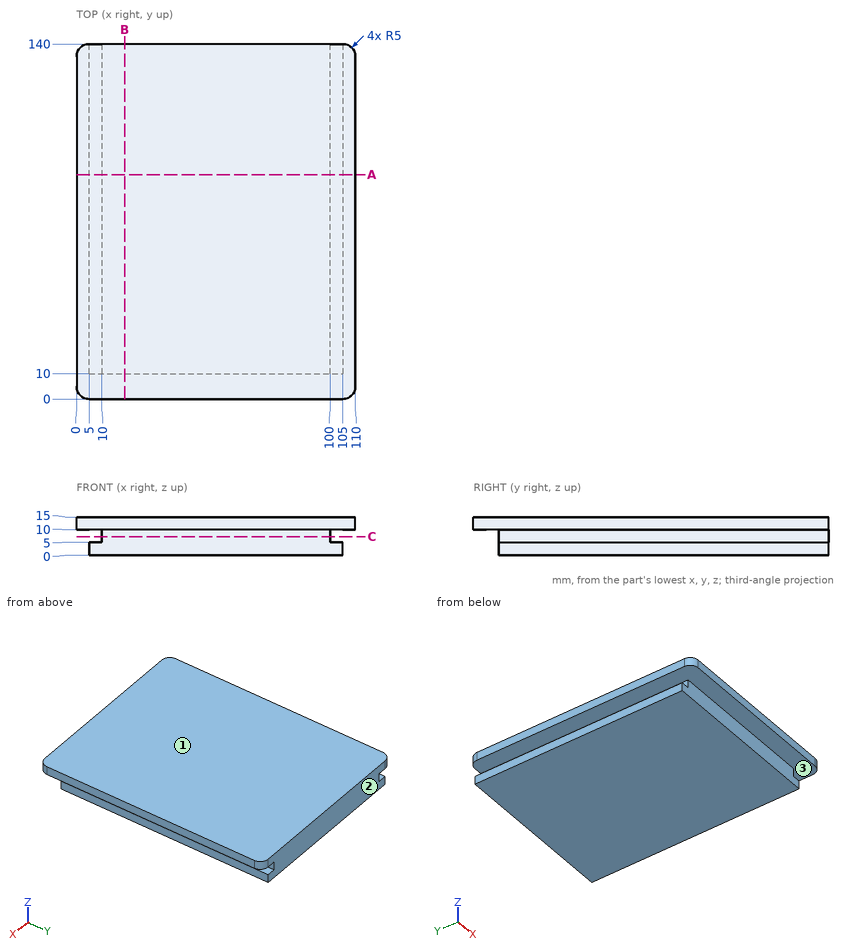
The figure shows three views and two pictorial views of one solid part (mm, origin at its lowest corner). Answer the questions. Coordinates: 2 decimals unless noted, no trailing zeros. Loops run counter-clockwise (first coordinate to the right, second up) from the corner with the lowest first, then second, coordinate; pieces in that order, holes last. Notation, with made-up numbers: (47, 35.25) - (106, 35.25) arc R12 ccw to (106, 57.25) - close; hole circle Ø9 at (55.5, 10). An arc over 180 degrees is marked (long way). Use a Markdown table: item, result. Add a question column.
1) The mould has two halves that part along Z. Classify the marked faces 1, 2 and 3: released by +Z, released by -Z, zero draft, split by the parting line, or undercut.
2) The part is cut by section C-C, the plane z = 7.25. Give the vertices of the cut face in (x, y).
3) Given pin 1 (2.5 mm diameter, centred on y = 85, z = 7.5, fed in from -X); pin 2 (4 mm diameter, centred on y = 68.5, z = 3.5, fed in from -X); pin 3 (1.5 mm diameter, centred on y = 67.5, z = 7, fed in from +X), each flat-ended and moving along its own axis, determine where each tip first touches the part or whether it passes through.
4) The part is cut by section B-B, the plane x = 19. Give the vertices of the cut face in (y, z), and give its area (3 significant figures).
5) The part is cut by section A-A, the plane y = 88.5. Give the vertices of the cut face in (x, z).
6) Find the intervals of material crossed by line 1 (Z direction, x = 7, y = 74.5); line 2 (X direction, y = 11.5, z = 7); line 3 (Y direction, x = 60, z = 3), in increasing order.
Here are the results:
| question | item | result |
|---|---|---|
| 1 | face 1 | released by +Z |
| 1 | face 2 | zero draft |
| 1 | face 3 | undercut |
| 2 | outline | (10, 10) - (100, 10) - (100, 140) - (10, 140) - close |
| 3 | pin 1 | stops at x = 10 |
| 3 | pin 2 | stops at x = 5 |
| 3 | pin 3 | stops at x = 100 |
| 4 | outline | (0, 10) - (10, 10) - (10, 0) - (140, 0) - (140, 15) - (0, 15) - close |
| 4 | area | 2,000 mm^2 |
| 5 | outline | (0, 10) - (10, 10) - (10, 5) - (5, 5) - (5, 0) - (105, 0) - (105, 5) - (100, 5) - (100, 10) - (110, 10) - (110, 15) - (0, 15) - close |
| 6 | line 1 | z = 0 to 5, 10 to 15 |
| 6 | line 2 | x = 10 to 100 |
| 6 | line 3 | y = 10 to 140 |
